Check sheet for the modelled part. Datum: model origin and axes. Units: mm. Round coordinates to 2 decimals unless told otherwise and drop trailing zeros. Order: outer loops, then holes, each group sorted by start corner. A loop starts at its lowest first (then second) coordinate and runs counter-clockwise, first axis right, second up. Notation, with made-up numbers: (16.5, -39.5) -> (33.5, -39.5) arc R11 ccw to (33.5, -25.5) -> close; hole circle Ø2 at (-35.5, 1.5). An arc over 180 degrees is marked (long way). Answer in a Markdown table with one row per item.
from build123d import *

# Parameters (mm, degrees)
SKETCH1_W           = 60
SKETCH1_H           = 126
BOSS_EXTRUDE1_DEPTH = 3
SKETCH2_R           = 2.5
CUT_EXTRUDE1_DEPTH  = 5


with BuildPart() as part:
    # Sketch1 → Boss-Extrude1 (new body)
    with BuildSketch(Plane(origin=(0, 0, 0), x_dir=(1, 0, 0), z_dir=(0, 1, 0))):
        Rectangle(SKETCH1_W, SKETCH1_H)
    extrude(amount=BOSS_EXTRUDE1_DEPTH)

    # Sketch2 → Cut-Extrude1 (cut)
    with BuildSketch(Plane(origin=(0, 3, 0), x_dir=(1, 0, 0), z_dir=(0, 1, 0))):
        with Locations((0, -58)):
            Circle(SKETCH2_R)
        with Locations((20, -58)):
            Circle(SKETCH2_R)
        with Locations((-20, -58)):
            Circle(SKETCH2_R)
        with Locations((20, 58)):
            Circle(SKETCH2_R)
        with Locations((0, 58)):
            Circle(SKETCH2_R)
        with Locations((-20, 58)):
            Circle(SKETCH2_R)
        Circle(SKETCH2_R)
    extrude(amount=-CUT_EXTRUDE1_DEPTH, mode=Mode.SUBTRACT)


solid = part.part
Item 1: Scan lines: line 1 (X direction, y = 2.4, z = 58); line 2 (Z direction, x = 20, y = 2); line 3 (Z direction, x = 0, y = 1.4). Record each from-to range of solid material in increasing order. Write a range as [from, to].
Result sheet:
| item | result |
|---|---|
| line 1 | x = [-30, -22.5], [-17.5, -2.5], [2.5, 17.5], [22.5, 30] |
| line 2 | z = [-63, -60.5], [-55.5, 55.5], [60.5, 63] |
| line 3 | z = [-63, -60.5], [-55.5, -2.5], [2.5, 55.5], [60.5, 63] |
Item 2: Mould release check, pull along Z, two halves, no side actions. Record for faces 1 (the flat face through (0, 1, -63)), 2 (the flat face through (0, 1, 63)), 3 (the cylindrical face through (-22.5, 1.5, -58.1)): pulls with the +Z half, pulls with the -Z half, needs draft (parallel to the pull), parting line crosses it, or undercut.
Result sheet:
| item | result |
|---|---|
| face 1 | pulls with the -Z half |
| face 2 | pulls with the +Z half |
| face 3 | undercut |
Item 3: Cross-section at A-A (x = -20). Record the boundary of the cut face in (y, z), and give its area (3 significant figures).
Result sheet:
| item | result |
|---|---|
| outline | (0, -63) -> (3, -63) -> (3, -60.5) -> (0, -60.5) -> close; (0, -55.5) -> (3, -55.5) -> (3, 55.5) -> (0, 55.5) -> close; (0, 60.5) -> (3, 60.5) -> (3, 63) -> (0, 63) -> close |
| area | 348 mm^2 |
Item 4: Cross-section at B-B (z = -58). Record the boundary of the cut face in (x, y).
Result sheet:
| item | result |
|---|---|
| outline | (-30, 0) -> (-22.5, 0) -> (-22.5, 3) -> (-30, 3) -> close; (-17.5, 0) -> (-2.5, 0) -> (-2.5, 3) -> (-17.5, 3) -> close; (2.5, 0) -> (17.5, 0) -> (17.5, 3) -> (2.5, 3) -> close; (22.5, 0) -> (30, 0) -> (30, 3) -> (22.5, 3) -> close |
Item 5: Cross-section at C-C (x = 0). Record the boundary of the cut face in (y, z).
Result sheet:
| item | result |
|---|---|
| outline | (0, -63) -> (3, -63) -> (3, -60.5) -> (0, -60.5) -> close; (0, -55.5) -> (3, -55.5) -> (3, -2.5) -> (0, -2.5) -> close; (0, 2.5) -> (3, 2.5) -> (3, 55.5) -> (0, 55.5) -> close; (0, 60.5) -> (3, 60.5) -> (3, 63) -> (0, 63) -> close |
Item 6: Cross-section at D-D (y = 1.1). Record the boundary of the cut face in (x, z).
Result sheet:
| item | result |
|---|---|
| outline | (-30, -63) -> (30, -63) -> (30, 63) -> (-30, 63) -> close; hole circle Ø5 at (-20, -58); hole circle Ø5 at (-20, 58); hole circle Ø5 at (0, -58); hole circle Ø5 at (0, 0); hole circle Ø5 at (0, 58); hole circle Ø5 at (20, -58); hole circle Ø5 at (20, 58) |
Item 7: Depth check by flat-ended pin: P1, Ø1.5, axis at x = -13.5, z = -19.5, coming from the -Y side. Enter the tip coordinate at first touch or a pass-through.
Result sheet:
| item | result |
|---|---|
| P1 | stops at y = 0 |
